Design review of the part built by this model. Coordinates are the model's own, in mm. Face numbers are marked on the shaded views. Coordinates: 2 decimals unless noted, no trailing zeros. Loops run counter-clockwise (first coordinate to the right, second up) from the corner with the lowest first, then second, coordinate; pieces in that order, holes last. Notation, with made-up numbers: (16.5, -30) -> (63.5, -30) arc R23 cw to (63.5, 2) -> close; hole circle Ø9 at (31, -22.75). An arc over 180 degrees is marked (long way). Use a Markdown table: item, result. Add a question column.
Q1. Take a section at C-C on z = 1.5. Write out the cut boundary in (x, y), plus the area to 3 significant figures.
Q2. Take a section at B-B on x = 0. Write out the cut boundary in (y, z).
Q3. Draft analysis for pull direction Y (two halves, no side actions). For the marked faces 1, 2, 3 and 4, state which applies: pulls with the +Y half, pulls with the -Y half, needs draft (parallel to the pull), parting line crosses it, or undercut.
Q4. For probe 1 along Y at (x, z) = (0, 2.5); probe 2 along Y at (x, z) = (0.5, 3.75); probe 3 along X at (y, z) = (-33, 3.75), list the stretches that pass through material, from the lowest coordinate up.
Q5. Take a section at A-A on y = -12.5. Write out the cut boundary in (x, z), plus the area to 3 significant figures.
from build123d import *

# Parameters (mm, degrees)
F0_W     = 15
F0_H     = 75
F0_R     = 2.6
F0_R_2   = 2.1
F1_DEPTH = 6
F2_R     = 5
F3_SIZE  = 0.5


with BuildPart() as f1:
    # F0 (on Top) → F1 (new body)
    with BuildSketch(Plane.XY):
        Rectangle(F0_W, F0_H)
        with Locations((-0.0689222117, -29.5514707496)):
            Circle(F0_R, mode=Mode.SUBTRACT)
        with Locations((-0.0689222117, -12.5)):
            Circle(F0_R_2, mode=Mode.SUBTRACT)
        with Locations((0, 12.5)):
            Circle(F0_R_2, mode=Mode.SUBTRACT)
        with Locations((0, 29.4484889938)):
            Circle(F0_R, mode=Mode.SUBTRACT)
    extrude(amount=F1_DEPTH)

    # F2
    f2_edges = [f1.edges().sort_by_distance(p)[0] for p in [
        (-7.5, 37.5, 3),
        (7.5, 37.5, 3),
        (-7.5, -37.5, 3),
        (7.5, -37.5, 3),
    ]]
    fillet(f2_edges, radius=F2_R)

    # F3
    f3_edges = [f1.edges().sort_by_distance(p)[0] for p in [
        (-7.5, 0, 6),
        (7.5, 0, 6),
        (6.035534, 36.035534, 6),
        (0, 37.5, 6),
        (-6.035534, 36.035534, 6),
        (-6.035534, -36.035534, 6),
        (0, -37.5, 6),
        (6.035534, -36.035534, 6),
        (-6.035534, 36.035534, 0),
        (0, 37.5, 0),
        (6.035534, 36.035534, 0),
        (7.5, 0, 0),
        (-7.5, 0, 0),
        (-6.035534, -36.035534, 0),
        (0, -37.5, 0),
        (6.035534, -36.035534, 0),
    ]]
    chamfer(f3_edges, length=F3_SIZE)


solid = f1.part
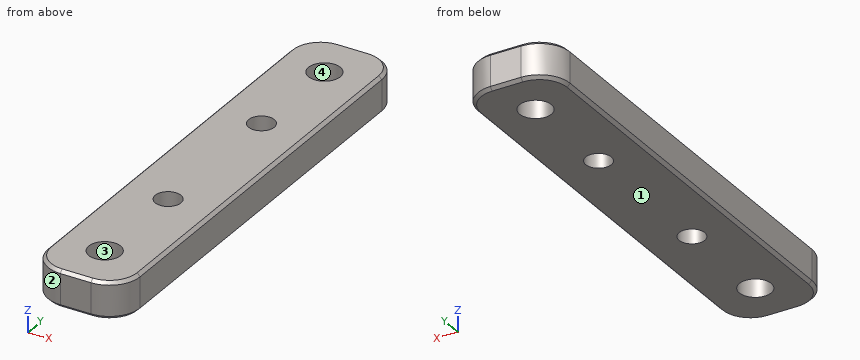
Answer list:
| question | item | result |
|---|---|---|
| 1 | outline | (-7.5, -32.5) arc R5 ccw to (-2.5, -37.5) -> (2.5, -37.5) arc R5 ccw to (7.5, -32.5) -> (7.5, 32.5) arc R5 ccw to (2.5, 37.5) -> (-2.5, 37.5) arc R5 ccw to (-7.5, 32.5) -> close; hole circle Ø5.2 at (-0.07, -29.55); hole circle Ø5.2 at (0, 29.45); hole circle Ø4.2 at (-0.07, -12.5); hole circle Ø4.2 at (0, 12.5) |
| 1 | area | 1,030 mm² |
| 2 | outline | (-37.5, 0.5) -> (-37, 0) -> (-32.15, 0) -> (-32.15, 6) -> (-37, 6) -> (-37.5, 5.5) -> close; (-26.95, 0) -> (-14.6, 0) -> (-14.6, 6) -> (-26.95, 6) -> close; (-10.4, 0) -> (10.4, 0) -> (10.4, 6) -> (-10.4, 6) -> close; (14.6, 0) -> (26.85, 0) -> (26.85, 6) -> (14.6, 6) -> close; (32.05, 0) -> (37, 0) -> (37.5, 0.5) -> (37.5, 5.5) -> (37, 6) -> (32.05, 6) -> close |
| 3 | face 1 | needs draft |
| 3 | face 2 | pulls with the -Y half |
| 3 | face 3 | undercut |
| 3 | face 4 | undercut |
| 4 | probe 1 | -37.5 to -32.15, -26.95 to -14.6, -10.4 to 10.4, 14.6 to 26.85, 32.05 to 37.5 |
| 4 | probe 2 | -37.5 to -32.09, -27.01 to -14.52, -10.48 to 10.46, 14.54 to 26.9, 32 to 37.5 |
| 4 | probe 3 | -7.47 to 7.47 |
| 5 | outline | (-7.5, 0.5) -> (-7, 0) -> (-2.17, 0) -> (-2.17, 6) -> (-7, 6) -> (-7.5, 5.5) -> close; (2.03, 0) -> (7, 0) -> (7.5, 0.5) -> (7.5, 5.5) -> (7, 6) -> (2.03, 6) -> close |
| 5 | area | 64.3 mm² |
